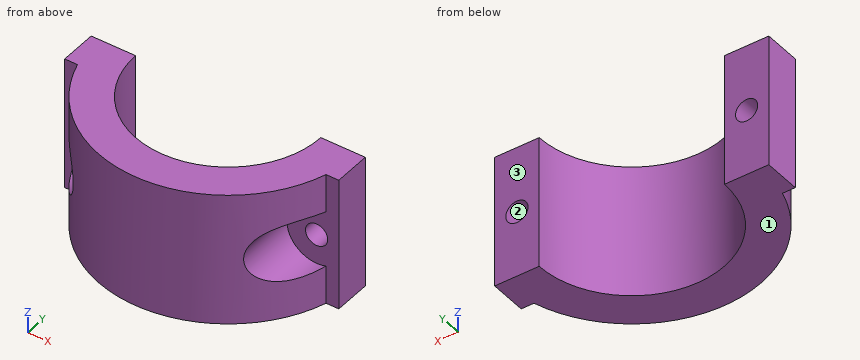
Autodesk Inventor part; units mm, degrees
ref_plane "YZ Plane" through (0, 0, 0) normal (1, 0, 0) x (0, 1, 0)
ref_plane "XZ Plane" through (0, 0, 0) normal (0, 1, 0) x (-1, 0, 0)
ref_plane "XY Plane" through (0, 0, 0) normal (0, 0, 1) x (1, 0, 0)
sketch "Sketch1" plane through (0, 0, 0) normal (0, 0, 1) x (1, 0, 0)
  arc A0 (-12.5, 0) -> (12.5, 0) centre (0, 0) ccw
  arc A1 (-16.7705, -5) -> (16.7705, -5) centre (0, 0) ccw
  line L0 (-16.5, 0) -> (-18.5, 0)
  line L1 (-18.5, 0) -> (-18.5, -5)
  line L2 (-18.5, -5) -> (-16.7705, -5)
  line L3 (16.5, 0) -> (18.5, 0)
  line L4 (18.5, 0) -> (18.5, -5)
  line L5 (18.5, -5) -> (16.7705, -5)
  line L6 (-16.5, 0) -> (-12.5, 0)
  line L7 (12.5, 0) -> (16.5, 0)
  point P0 (-17.5, 0)
  dimension "d0" = 25
  dimension "d2" = 5
  dimension "d3" = 2
  dimension "d4" = 5
  dimension "d22" = 6
extrude "Extrusion1" add sketch "Sketch1" along normal blind 18
sketch "Sketch2" plane through (-18.5, 0, 0) normal (0, 1, 0) x (1, 0, 0)
  circle A0 centre (3, -9) radius 1.5
  circle A1 centre (34, -9) radius 1.5
  line L0 (6, 0) -> (0, 0)
  line L1 (37, 0) -> (31, 0)
  line L2 (37, 0) -> (37, -18)
  line L3 (0, 0) -> (0, -18)
  line L4 (6, 0) -> (6, -18)
  line L5 (31, 0) -> (31, -18)
  point P0 (18.5, 0)
  dimension "d8" = 3
  dimension "d9" = 3
  dimension "d10" = 9
  dimension "d11" = 9
  dimension "d16" = 3
  dimension "d17" = 3
extrude "Extrusion2" cut sketch "Sketch2" against normal blind 18
sketch "Sketch3" plane through (-18.5, -5, 0) normal (0, -1, 0) x (1, 0, 0)
  circle A0 centre (3, 9) radius 1.5
  circle A1 centre (3, 9) radius 4
  circle A2 centre (34, 9) radius 1.5
  circle A3 centre (34, 9) radius 4
  point P0 (18.5, 0)
  dimension "d18" = 8
  dimension "d19" = 8
extrude "Extrusion3" cut sketch "Sketch3" along normal blind 10
properties part number "Clamp_Mount"
Part model, mm, in its own coordinate system. Face numbers are marked on the shaded views. Give positions to 0.01 mm unless a question says otherwise; leave off trailing zeros. Loops run counter-clockwise (first coordinate to the right, second up) from the corner with the lowest first, then second, coordinate; pieces in that order, holes last. Notation, with made-up numbers: M 47.25,89 L 57.25,89 A16 ccw 57.25,115 Z; hole C 43,64 d10. An arc over 180 degrees is marked long. Put each result on its own line as item: value. Start each with the question number.
1) Saw through at A-A (z = 9). List the corners of the cut face in (x, y).
2) Flat gauge pins, fed straight in: pin 1 (8 mm diameter, centred on x = -5, z = 13, fed in from -Y); pin 2 (7 mm diameter, centred on x = 15.5, z = 9, fed in from -Y); pin 3 (1 mm diameter, centred on y = -15.5, z = 9.5, fed in from -X). Where does each tip first touch, or does it go through?
3) Saw through at D-D (x = 15.5). List the corners of the cut face in (y, z).
4) Saw through at B-B (z = 15). List the corners of the cut face in (x, y), then the cut area to 3 significant figures.
5) Saw through at C-C (y = -10.5). List the corners of the cut face in (x, z), then the cut area to 3 significant figures.
6) Probe probe 1 along Z at (x, y) = (-15.5, -2.35); probe 2 along X at (y, z) = (-7.5, 14); probe 3 along Z at (x, y) = (-15.5, -7). List the from-to ranges inside material, lowest first.
7) Pull direction Z, two halves, no side cores. Call the marked faces 1, 2 and 3: +Z half, -Z half, draft (parallel to the pull), parting line (faces both ways), or undercut.
Numbers:
1. outline: M -18.5,-5 L -17,-5 L -17,0 L -18.5,0 Z; M -14,-5 L -11.5,-5 L -11.5,-13.19 A17.5 ccw 11.5,-13.19 L 11.5,-5 L 14,-5 L 14,0 L 12.5,0 A12.5 cw -12.5,0 L -14,0 Z; M 17,-5 L 18.5,-5 L 18.5,0 L 17,0 Z
2. pin 1: y = -17.47
2. pin 2: y = -5
2. pin 3: x = -9.01
3. outline: M -8.12,0 L 0,0 L 0,7.5 L -5,7.5 L -5,5 L -8.12,5 Z; M -8.12,13 L -5,13 L -5,10.5 L 0,10.5 L 0,18 L -8.12,18 Z
4. outline: M -18.5,-5 L -16.77,-5 A17.5 ccw 16.77,-5 L 18.5,-5 L 18.5,0 L 12.5,0 A12.5 cw -12.5,0 L -18.5,0 Z
4. area: 248 mm^2
5. outline: M -14,0 L -6.78,0 L -6.78,18 L -14,18 L -14,12.71 A4 cw -14,5.29 Z; M 6.78,0 L 14,0 L 14,5.29 A4 cw 14,12.71 L 14,18 L 6.78,18 Z
5. area: 233 mm^2
6. probe 1: 0 to 7.5, 10.5 to 18
6. probe 2: -15.81 to -10, 10 to 15.81
6. probe 3: 0 to 5, 13 to 18
7. face 1: -Z half
7. face 2: undercut
7. face 3: draft
